For this review, take the finished solid that the model builds, in its own axes (mm). A direction names the side the tool comes from. Give positions to 0.01 mm unless a question says otherwise; leave off trailing zeros. Order: outer loops, then holes, each group sorted by start corner. A loop starts at its lowest first (then second) coordinate and runs counter-clockwise, first axis right, second up. Notation, with made-up numbers: M 43,-26.75 L 94,-26.75 A13 ccw 94,-14.75 Z; hole C 67,-2.5 d3. An arc over 180 degrees is marked long. Answer as CSV lines item,"result". Start each with the question number.
1. Mouldability with a two-part tool opening along X and no side actions: class faces 1 (the flat face through (86, 1, -3.81)), 2 (the cylindrical face through (2.29, 33.68, -1.88)), 3 (the flat face through (108.53, 22.877, -1.932)), 4 (the flat face through (13.509, 16, -2)) as pulls with the +X half, pulls with the -X half, needs draft (parallel to the pull), parting line crosses it, or undercut.
2. We need section A-A, the plane y = 7. State how many separate pieces and enclosed holes the cut face has, and give its area (3 significant figures).
3. We need section C-C, the plane z = -2.15. Give the boundary of the cut face in (x, y), and give its area (3 significant figures).
4. Machinability: for faces 5 (the flat face through (83, 18, -1.27)), 6 (the flat face through (109.11, 17.76, -0.64)), 7 (the flat face through (100.262, 25.319, -1.932)), 8 (the cylindrical face through (17.825, 31.521, -2.504)), which of the approach directions +Z, -Z, +X, -X, +Y, -Y give a long, thin tool a straight path to every point of the face, cutting with its end or side? Answer none if there is none.
5. Clearance check with flat-ended pins moving along their axes: P1, Ø9.5, axis at x = 80.5, y = 23.5, coming from the -Z side; P2, Ø3, axis at y = 12.5, z = -1, coming from the +X side; P3, Ø10, axis at x = 94.5, y = 24, coming from the +Z side; P4, Ø3, axis at x = 96.5, z = -2.5, coming from the +Y side. State where each tip first meets the part, or that it passes through.
6. For line 1 along X through (y, z) = (15.5, -1.4); line 2 along Y through (x, z) = (66, -3.2); line 3 along Y through (x, z) = (89.5, -1.2), list the stretches that pass through material, from the lowest coordinate up.
7. We need section B-B, the plane x = 86. Give the boundary of the cut face in (y, z).
from build123d import *

# Parameters (mm, degrees)
EXTRUDE1_DEPTH          = 5.08
EXTRUDE2_DEPTH          = 1.27
EXTRUDE3_DEPTH          = 3.81
SKETCH1_5_W             = 4.91012523
SKETCH1_5_H             = 32.245498845
EXTRUDE4_DEPTH          = 3.81
FILLET2_R               = 1.27
FILLET3_R               = 1.27
CUT_EXTRUDE1_DEPTH      = 123.54722299
CUT_EXTRUDE1_DEPTH_BACK = 123.54722299


with BuildPart() as part:
    # Sketch1 → Extrude1 (new, symmetric)
    with BuildSketch(Plane.XY):
        with BuildLine():
            Line((55.053954756, 23.223525864), (55.053954756, 28.234899079))
            ThreePointArc((55.053954756, 28.234899079), (52.822108428, 33.623052752), (47.433954756, 35.854899079))
            Line((47.433954756, 35.854899079), (7.62, 35.854899079))
            ThreePointArc((7.62, 35.854899079), (2.231846327, 33.623052752), (0, 28.234899079))
            Line((0, 28.234899079), (0, -28.234899079))
            ThreePointArc((0, -28.234899079), (2.231846327, -33.623052752), (7.62, -35.854899079))
            Line((7.62, -35.854899079), (47.433954756, -35.854899079))
            ThreePointArc((47.433954756, -35.854899079), (52.822108428, -33.623052752), (55.053954756, -28.234899079))
            Line((55.053954756, -28.234899079), (55.053954756, -23.223525864))
            Line((55.053954756, -23.223525864), (55.053954756, -19.324782682))
            Line((55.053954756, -19.324782682), (55.053954756, -16.240810389))
            Line((55.053954756, -16.240810389), (55.053954756, -5.571934871))
            Line((55.053954756, -5.571934871), (55.053954756, -2.359181621))
            Line((55.053954756, -2.359181621), (55.053954756, 2.359181621))
            Line((55.053954756, 2.359181621), (55.053954756, 5.571934871))
            Line((55.053954756, 5.571934871), (55.053954756, 16.240810389))
            Line((55.053954756, 16.240810389), (55.053954756, 19.324782682))
            Line((55.053954756, 19.324782682), (55.053954756, 23.223525864))
        make_face()
        with BuildLine():
            ThreePointArc((16.048576777, 32.245498845), (17.844628001, 31.501550069), (18.588576777, 29.705498845))
            Line((18.588576777, 29.705498845), (18.588576777, 27.618036038))
            Line((18.588576777, 27.618036038), (41.829183295, 27.618036038))
            ThreePointArc((41.829183295, 27.618036038), (46.643426698, 25.623911128), (48.637551607, 20.809667725))
            Line((48.637551607, 20.809667725), (48.637551607, -20.809667725))
            ThreePointArc((48.637551607, -20.809667725), (46.643426698, -25.623911128), (41.829183295, -27.618036038))
            Line((41.829183295, -27.618036038), (18.588576777, -27.618036038))
            Line((18.588576777, -27.618036038), (18.588576777, -29.705498845))
            ThreePointArc((18.588576777, -29.705498845), (17.844628001, -31.501550069), (16.048576777, -32.245498845))
            Line((16.048576777, -32.245498845), (13.508576777, -32.245498845))
            Line((13.508576777, -32.245498845), (8.598451547, -32.245498845))
            Line((8.598451547, -32.245498845), (6.058451547, -32.245498845))
            ThreePointArc((6.058451547, -32.245498845), (4.262400322, -31.501550069), (3.518451547, -29.705498845))
            Line((3.518451547, -29.705498845), (3.518451547, 29.705498845))
            ThreePointArc((3.518451547, 29.705498845), (4.262400322, 31.501550069), (6.058451547, 32.245498845))
            Line((6.058451547, 32.245498845), (8.598451547, 32.245498845))
            Line((8.598451547, 32.245498845), (13.508576777, 32.245498845))
            Line((13.508576777, 32.245498845), (16.048576777, 32.245498845))
        make_face(mode=Mode.SUBTRACT)
    extrude(amount=EXTRUDE1_DEPTH, both=True)

    # Sketch1<3> → Extrude2 (add, symmetric)
    with BuildSketch(Plane.XY):
        Polygon((110.911701022, 19.324782682), (55.053954756, 19.324782682), (55.053954756, 16.240810389), (107.354901489, 16.240810389), align=None)
        Polygon((114.44157437, -2.359181621), (55.053954756, -2.359181621), (55.053954756, -5.571934871), (107.985089149, -5.571934871), align=None)
        Polygon((107.985089149, 5.571934871), (55.053954756, 5.571934871), (55.053954756, 2.359181621), (114.44157437, 2.359181621), align=None)
        Polygon((107.354901489, -16.240810389), (55.053954756, -16.240810389), (55.053954756, -19.324782682), (110.911701022, -19.324782682), align=None)
    extrude(amount=EXTRUDE2_DEPTH, both=True)

    # Sketch1<4> → Extrude3 (add, symmetric)
    with BuildSketch(Plane.XY):
        with BuildLine():
            Line((99.519849351, 23.223525864), (55.053954756, 23.223525864))
            Line((55.053954756, 23.223525864), (55.053954756, 19.324782682))
            Line((55.053954756, 19.324782682), (110.911701022, 19.324782682))
            ThreePointArc((110.911701022, 19.324782682), (111.174479609, 19.893330482), (110.922452685, 20.466725298))
            Line((110.922452685, 20.466725298), (106.069134127, 25.355454719))
            ThreePointArc((106.069134127, 25.355454719), (104.150057648, 26.85581949), (101.918508412, 27.832618847))
            ThreePointArc((101.918508412, 27.832618847), (101.356567079, 27.780652221), (100.984486575, 27.356347272))
            Line((100.984486575, 27.356347272), (99.519849351, 23.223525864))
        make_face()
        Polygon((114.44157437, 2.359181621), (55.053954756, 2.359181621), (55.053954756, -2.359181621), (114.44157437, -2.359181621), (117.074513308, -1.049028675), (117.074513308, 1.049028675), align=None)
        with BuildLine():
            Line((55.053954756, -19.324782682), (55.053954756, -23.223525864))
            Line((55.053954756, -23.223525864), (99.519849351, -23.223525864))
            Line((99.519849351, -23.223525864), (101.216749822, -28.011733127))
            ThreePointArc((101.216749822, -28.011733127), (103.835645626, -27.035617331), (106.069134127, -25.355454719))
            Line((106.069134127, -25.355454719), (110.922452685, -20.466725298))
            ThreePointArc((110.922452685, -20.466725298), (111.174479609, -19.893330482), (110.911701022, -19.324782682))
            Line((110.911701022, -19.324782682), (55.053954756, -19.324782682))
        make_face()
    extrude(amount=EXTRUDE3_DEPTH, both=True)

    # Sketch1<5> → Extrude4 (add, symmetric)
    with BuildSketch(Plane.XY):
        with BuildLine():
            Line((48.637551607, 0), (18.588576777, 0))
            Line((18.588576777, 0), (18.588576777, -27.618036038))
            Line((18.588576777, -27.618036038), (41.829183295, -27.618036038))
            ThreePointArc((41.829183295, -27.618036038), (46.643426698, -25.623911128), (48.637551607, -20.809667725))
            Line((48.637551607, -20.809667725), (48.637551607, 0))
        make_face()
        with BuildLine():
            Line((18.588576777, 27.618036038), (18.588576777, 0))
            Line((18.588576777, 0), (48.637551607, 0))
            Line((48.637551607, 0), (48.637551607, 20.809667725))
            ThreePointArc((48.637551607, 20.809667725), (46.643426698, 25.623911128), (41.829183295, 27.618036038))
            Line((41.829183295, 27.618036038), (18.588576777, 27.618036038))
        make_face()
        with Locations((11.053514162, -16.122749423)):
            Rectangle(SKETCH1_5_W, SKETCH1_5_H)
        with Locations((11.053514162, 16.122749423)):
            Rectangle(SKETCH1_5_W, SKETCH1_5_H)
    extrude(amount=EXTRUDE4_DEPTH, both=True)

    # Fillet2
    fillet2_edges = [part.edges().sort_by_distance(p)[0] for p in [
        (30.208880036, -27.618036038, -3.81),
        (30.208880036, -27.618036038, 3.81),
        (46.643426698, -25.623911128, -3.81),
        (46.643426698, -25.623911128, 3.81),
        (48.637551607, 0, -3.81),
        (48.637551607, 0, 3.81),
        (46.643426698, 25.623911128, -3.81),
        (46.643426698, 25.623911128, 3.81),
        (30.208880036, 27.618036038, -3.81),
        (30.208880036, 27.618036038, 3.81),
    ]]
    fillet(fillet2_edges, radius=FILLET2_R - 0.0001)  # a hair under: the kernel refuses the full size

    # Fillet3
    fillet3_edges = [part.edges().sort_by_distance(p)[0] for p in [
        (2.231846327, 33.623052752, -5.08),
        (27.526977378, 35.854899079, -5.08),
        (52.822108428, 33.623052752, -5.08),
        (55.053954756, 0, -5.08),
        (52.822108428, -33.623052752, -5.08),
        (27.526977378, -35.854899079, -5.08),
        (2.231846327, -33.623052752, -5.08),
        (0, 0, -5.08),
        (0, 0, 5.08),
        (2.231846327, -33.623052752, 5.08),
        (27.526977378, -35.854899079, 5.08),
        (52.822108428, -33.623052752, 5.08),
        (55.053954756, 0, 5.08),
        (52.822108428, 33.623052752, 5.08),
        (27.526977378, 35.854899079, 5.08),
        (2.231846327, 33.623052752, 5.08),
    ]]
    fillet(fillet3_edges, radius=FILLET3_R - 0.0001)  # a hair under: the kernel refuses the full size

    # Sketch2 → Cut-Extrude1 (cut, two sides: drawn at the far end of the back side and taken through both)
    with BuildSketch(Plane(origin=(117.074513308, 0, 0), x_dir=(0, 0, -1), z_dir=(1, 0, 0)).offset(-CUT_EXTRUDE1_DEPTH_BACK)):
        Polygon((158.859018875, 0), (5.08, 0), (0, 0), (0, 35.854899079), (0, 189.633917954), (-235.763888228, -7.868830363), (-76.904869352, -197.502748317), align=None)
    extrude(amount=CUT_EXTRUDE1_DEPTH + CUT_EXTRUDE1_DEPTH_BACK, mode=Mode.SUBTRACT)


solid = part.part
Result set:
1,face 1,"needs draft"
1,face 2,"pulls with the -X half"
1,face 3,"pulls with the +X half"
1,face 4,"undercut"
2,separate pieces,"3"
2,enclosed holes,"0"
2,area,"183 mm2"
3,outline,"M 0,0 L 3.52,0 L 3.52,29.71 A2.54 cw 6.06,32.25 L 8.6,32.25 L 8.6,0 L 13.51,0 L 13.51,32.25 L 16.05,32.25 A2.54 cw 18.59,29.71 L 18.59,0 L 117.07,0 L 117.07,1.05 L 114.44,2.36 L 55.05,2.36 L 55.05,19.32 L 110.91,19.32 A0.76 ccw 110.92,20.47 L 106.07,25.36 A9.73 ccw 101.92,27.83 A0.76 ccw 100.98,27.36 L 99.52,23.22 L 55.05,23.22 L 55.05,28.23 A7.62 ccw 47.43,35.85 L 7.62,35.85 A7.62 ccw 0,28.23 Z"
3,area,"2,010 mm2"
4,face 5,"-Z, +X"
4,face 6,"+Z, -Z, +X"
4,face 7,"+Z, -Z, +Y"
4,face 8,"+Z, -Z, -Y"
5,P1,"z = -3.81"
5,P2,"x = 55.05"
5,P3,"z = 0"
5,P4,"y = 23.22"
6,line 1,"0 to 3.52, 8.6 to 13.51, 18.59 to 55.05"
6,line 2,"0 to 2.36, 19.32 to 23.22"
6,line 3,"0 to 5.57, 16.24 to 23.22"
7,outline,"M 0,-3.81 L 2.36,-3.81 L 2.36,-1.27 L 5.57,-1.27 L 5.57,0 L 0,0 Z; M 16.24,-1.27 L 19.32,-1.27 L 19.32,-3.81 L 23.22,-3.81 L 23.22,0 L 16.24,0 Z"
